The drawing under review shows one solid part. Ordinate dimensions are in mm from its lowest x, y, z. A direction names the side the tool comes from. Coordinates: 2 decimals unless noted, no trailing zeros. Write each loop counter-clockwise with the first axis right and the second up, starting at its lowest first coordinate (ties: lowest second). Pieces come first, ordered by that corner, then holes.
Q1. Clearance check with flat-ended pins moving along their axes: pin 1 Ø13 at (x, z) = (20, 14) entering from -Y; pin 2 Ø3 at (y, z) = (13, 36) entering from -X; pin 3 Ø1 at (x, y) = (6.5, 4) entering from +Z; pin 4 Ø1 at (y, z) = (8, 22.5) entering from +X. State where each tip first meets the part, or that it passes through.
Q2. Machinability: for the marked faces 1, 2, 3 and 4, which of the approach directions +Z, -Z, +X, -X, +Y, -Y give a long, thin tool a straight path to every point of the face, cutting with its end or side? Answer none if there is none.
Q3. Add section C-C, the plane z = 37. Give the boundary of the cut face in (x, y).
Q4. Add section A-A, the plane x = 4. Give the boundary of the cut face in (y, z).
Q5. Add section D-D, the plane y = 10. Give the number of separate pieces and of enclosed holes in the cut face, plus the area to 3 significant figures.
Q6. To check wall thickness, follow probe 1 along X at (y, z) = (10, 0.45); probe 2 along X at (y, z) = (1.75, 36); probe 3 along Y at (x, z) = (18, 31.5). State the ranges of each line that lie inside material, in increasing order.
Q7. The part is to be moulded in two halves that separate along Y. For the marked faces 5, 6, 7 and 8, say which applies: +Y half, -Y half, draft (parallel to the pull), parting line (faces both ways), or undercut.
Q8. Add section B-B, the plane y = 5.25. Give the boundary of the cut face in (x, z).
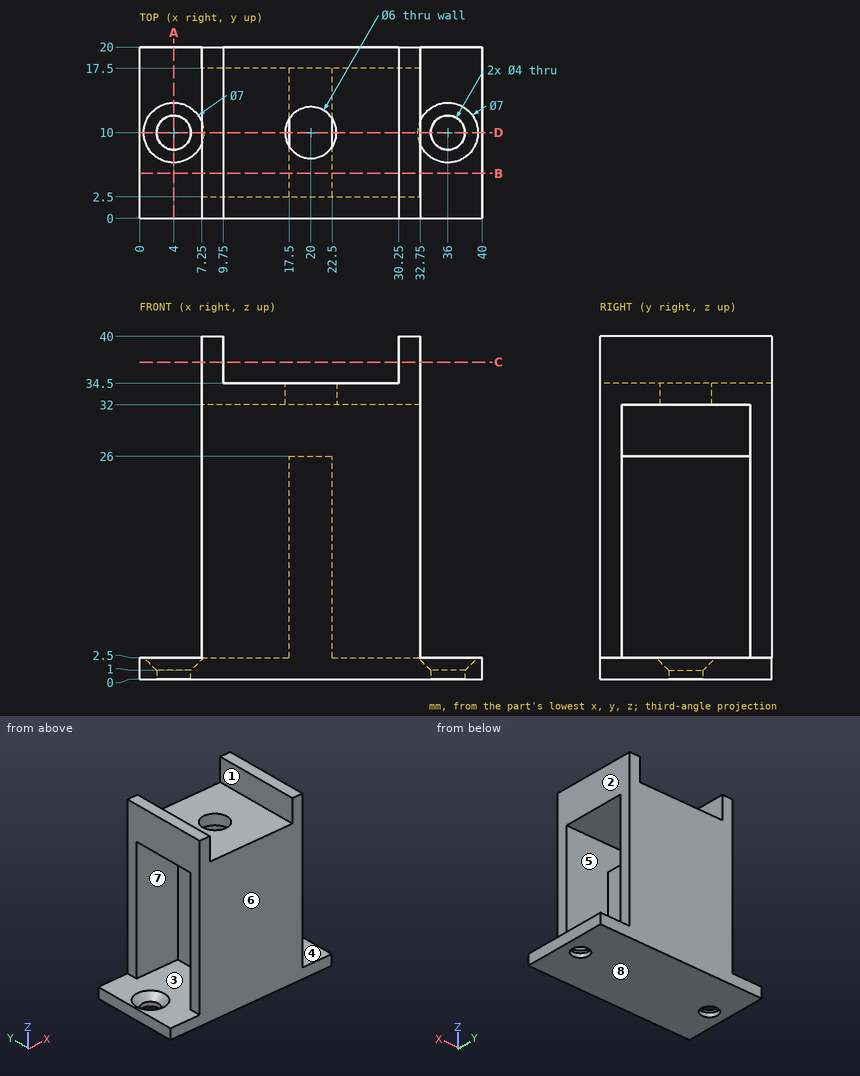
Here are the results:
1. pin 1: stops at y = 0
1. pin 2: stops at x = 7.25
1. pin 3: stops at z = 2.5
1. pin 4: stops at x = 22.5
2. face 1: +Z, +Y, -Y
2. face 2: +Z, +X, +Y, -Y
2. face 3: -X
2. face 4: +X
3. outline: (7.25, 0) - (9.75, 0) - (9.75, 20) - (7.25, 20) - close; (30.25, 0) - (32.75, 0) - (32.75, 20) - (30.25, 20) - close
4. outline: (0, 0) - (8, 0) - (8, 1) - (6.5, 2.5) - (0, 2.5) - close; (12, 0) - (20, 0) - (20, 2.5) - (13.5, 2.5) - (12, 1) - close
5. separate pieces: 5
5. enclosed holes: 0
5. area: 269 mm2
6. probe 1: x = 0 to 2, 6 to 34, 38 to 40
6. probe 2: x = 7.25 to 9.75, 30.25 to 32.75
6. probe 3: y = 0 to 2.5, 17.5 to 20
7. face 5: undercut
7. face 6: -Y half
7. face 7: undercut
7. face 8: draft
8. outline: (0, 0) - (40, 0) - (40, 2.5) - (22.5, 2.5) - (22.5, 26) - (17.5, 26) - (17.5, 2.5) - (0, 2.5) - close; (7.25, 32) - (32.75, 32) - (32.75, 40) - (30.25, 40) - (30.25, 34.5) - (9.75, 34.5) - (9.75, 40) - (7.25, 40) - close
